Source: CAD feature listing. Evaluate the final solid. Frame: model axes, mm. Face numbers are marked on the shaded views. A direction names the side the tool comes from. Coordinates: 2 decimals unless noted, no trailing zeros. Write each loop counter-clockwise with the first axis right and the second up, starting at its lowest first coordinate (ties: lowest second). Pieces come first, ordered by that corner, then holes. Notation, with made-up numbers: M 86.5,66 L 103.5,66 A18 cw 103.5,77 Z; hole C -11.75,-18.75 d1. An arc over 180 degrees is marked long. Write item = value, one per line. Start each with the question number.
1. Line query: line 1 along Z through (x, y) = (-79.5, -50); line 2 along X through (y, z) = (-80, 25.5); line 3 along Y through (x, z) = (-78.5, 40). Output: solid intervals per line, ascending.
2. Section query A-A (y = -62). Output: boundary loops of the cut face in (x, z), then the cut area to 3 significant figures.
3. Access query for the marked faces 1, 2 and 3. Directions: +Z, -Z, +X, -X, +Y, -Y. A direction counts if a zero-diameter tool reaches every point of the face in a straight line with its end or side. Return the directions, or none.
4. Section query B-B (x = -25.5). Output: boundary loops of the cut face in (y, z).
5. Pin query (flat end, axial travel): pin 1 Ø2 at (y, z) = (38.5, 20) entering from +X; pin 2 Ø10 at (y, z) = (0.5, 16) entering from -X; pin 3 Ø2 at (x, z) = (45, 42) entering from -Y. Return the tip coordinate at first contact, or that it passes through.
6. Section query C-C (z = 40). Output: boundary loops of the cut face in (x, y), then the cut area to 3 significant figures.
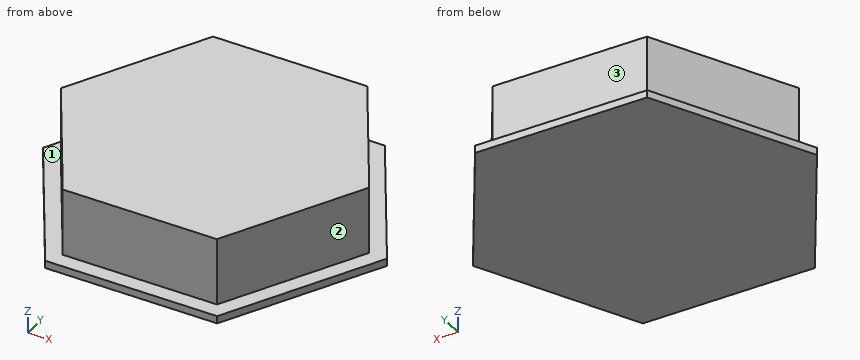
```python
from build123d import *

# Parameters (mm, degrees)
F1_DEPTH = 50
F3_DEPTH = 5


with BuildPart() as f1:
    # F0 (on Top) → F1 (new body)
    with BuildSketch(Plane.XY):
        Polygon((53.122164, -84.723289), (99.933603, 3.643499), (46.811438, 88.366788), (-53.122164, 84.723289), (-99.933603, -3.643499), (-46.811438, -88.366788), align=None)
    extrude(amount=F1_DEPTH)

    # F2 (on face) → F3 (join)
    with BuildSketch(Plane.XY):
        Polygon((-52.216758, -98.570506), (59.256183, -94.506292), (111.472941, 4.064214), (52.216758, 98.570506), (-59.256183, 94.506292), (-111.472941, -4.064214), align=None)
        Polygon((99.933603, 3.643499), (53.122164, -84.723289), (-46.811438, -88.366788), (-99.933603, -3.643499), (-53.122164, 84.723289), (46.811438, 88.366788), align=None, mode=Mode.SUBTRACT)
    extrude(amount=F3_DEPTH)


solid = f1.part
```
Results are:
q1.line_1 = 0 to 5
q1.line_2 = -52.06 to 55.62
q1.line_3 = -37.83 to 36.82
q2.outline = M -75.15,0 L 76.48,0 L 76.48,5 L 65.16,5 L 65.16,50 L -63.34,50 L -63.34,5 L -75.15,5 Z
q2.area = 6,540 mm^2
q3.face_1 = +Z
q3.face_2 = +Z, +X, -Y
q3.face_3 = +Z, -X, +Y
q4.outline = M -97.6,0 L 95.74,0 L 95.74,5 L 85.73,5 L 85.73,50 L -87.59,50 L -87.59,5 L -97.6,5 Z
q5.pin_1 = 78.71
q5.pin_2 = -99.93
q5.pin_3 = -85.06
q6.outline = M -99.93,-3.64 L -46.81,-88.37 L 53.12,-84.72 L 99.93,3.64 L 46.81,88.37 L -53.12,84.72 Z
q6.area = 26,000 mm^2
